Geometry: final body of the model. Coordinates: model frame, mm. Give positions to 0.01 mm unless a question says otherwise; leave off trailing zeros. Write each loop counter-clockwise with the first axis right and the second up, starting at its lowest first coordinate (ties: lowest second). Pieces come first, ordered by that corner, then holes. Notation, with made-up numbers: M 9.5,-10 L 23.5,-10 A13 cw 23.5,2 Z; hole C 22,-29 d9. An arc over 180 degrees is marked long. Answer as a JSON object with one key per item and string values.
from build123d import *

# Parameters (mm, degrees)
SKETCH_1_W          = 18
SKETCH_1_H          = 130
SKETCH_1_W_2        = 5
SKETCH_1_H_2        = 2
SKETCH_1_H_3        = 3
EXTRUDE_1_DEPTH     = 1.05
SKETCH_5_R          = 0.5
CUT_EXTRUDE_3_DEPTH = 69.625141166
SKETCH_2_W          = 1.05
SKETCH_2_H          = 25.1
CUT_EXTRUDE_1_DEPTH = 10
SKETCH_6_R          = 0.5
CUT_EXTRUDE_4_DEPTH = 69.625141166
CUT_EXTRUDE_5_DEPTH = 69.625141166
CUT_EXTRUDE_6_DEPTH = 69.625141166


with BuildPart() as part:
    # 草图1 → 凸台-拉伸1 (new, symmetric)
    with BuildSketch(Plane.XY):
        Rectangle(SKETCH_1_W, SKETCH_1_H)
        with Locations((-2.5, 66)):
            Rectangle(SKETCH_1_W_2, SKETCH_1_H_2)
        with Locations((2.5, 66)):
            Rectangle(SKETCH_1_W_2, SKETCH_1_H_2)
        with Locations((2.5, -66.5)):
            Rectangle(SKETCH_1_W_2, SKETCH_1_H_3)
        with Locations((-2.5, -66.5)):
            Rectangle(SKETCH_1_W_2, SKETCH_1_H_3)
    extrude(amount=EXTRUDE_1_DEPTH, both=True)

    # 草图5 → 切除-拉伸3 (cut, through all)
    with BuildSketch(Plane.XY.offset(1.05)):
        with Locations((5.353553391, 65.353553391)):
            Circle(SKETCH_5_R)
        with Locations((-5.353553391, 65.353553391)):
            Circle(SKETCH_5_R)
        with Locations((5.353553391, -65.353553391)):
            Circle(SKETCH_5_R)
        with Locations((-5.353553391, -65.353553391)):
            Circle(SKETCH_5_R)
    extrude(amount=-CUT_EXTRUDE_3_DEPTH, mode=Mode.SUBTRACT)

    # 草图2 → 切除-拉伸1 (cut)
    with BuildSketch(Plane.XY.offset(1.05)):
        with Locations((0.525, 37.5)):
            Rectangle(SKETCH_2_W, SKETCH_2_H)
        with Locations((-0.525, 37.5)):
            Rectangle(SKETCH_2_W, SKETCH_2_H)
        with Locations((0.525, -37.5)):
            Rectangle(SKETCH_2_W, SKETCH_2_H)
        with Locations((-0.525, -37.5)):
            Rectangle(SKETCH_2_W, SKETCH_2_H)
    extrude(amount=-CUT_EXTRUDE_1_DEPTH, mode=Mode.SUBTRACT)

    # 草图6 → 切除-拉伸4 (cut, through all)
    with BuildSketch(Plane.XY.offset(1.05)):
        with Locations((0.696446609, 49.696446609)):
            Circle(SKETCH_6_R)
        with Locations((-0.696446609, 49.696446609)):
            Circle(SKETCH_6_R)
        with Locations((0.696446609, 25.303553391)):
            Circle(SKETCH_6_R)
        with Locations((-0.696446609, 25.303553391)):
            Circle(SKETCH_6_R)
    cut_extrude_4 = extrude(amount=-CUT_EXTRUDE_4_DEPTH, mode=Mode.SUBTRACT)

    # 镜向1: 切除-拉伸4 across plane
    add(cut_extrude_4.mirror(Plane.ZX), mode=Mode.SUBTRACT)

    # 草图4 → 切除-拉伸5 (cut, through all)
    with BuildSketch(Plane.XY.offset(1.05)):
        with BuildLine():
            Line((6.2, 55), (6.2, 35))
            ThreePointArc((6.2, 35), (5, 33.8), (3.8, 35))
            Line((3.8, 35), (3.8, 55))
            ThreePointArc((3.8, 55), (5, 56.2), (6.2, 55))
        make_face()
        with BuildLine():
            Line((6.2, 25), (6.2, 5))
            ThreePointArc((6.2, 5), (5, 3.8), (3.8, 5))
            Line((3.8, 5), (3.8, 25))
            ThreePointArc((3.8, 25), (5, 26.2), (6.2, 25))
        make_face()
        with BuildLine():
            Line((6.2, -5), (6.2, -25))
            ThreePointArc((6.2, -25), (5, -26.2), (3.8, -25))
            Line((3.8, -25), (3.8, -5))
            ThreePointArc((3.8, -5), (5, -3.8), (6.2, -5))
        make_face()
        with BuildLine():
            Line((3.8, -55), (3.8, -35))
            ThreePointArc((3.8, -35), (5, -33.8), (6.2, -35))
            Line((6.2, -35), (6.2, -55))
            ThreePointArc((6.2, -55), (5, -56.2), (3.8, -55))
        make_face()
    cut_extrude_5 = extrude(amount=-CUT_EXTRUDE_5_DEPTH, mode=Mode.SUBTRACT)

    # 镜向2: 切除-拉伸5 across plane
    add(cut_extrude_5.mirror(Plane(origin=(0, 0, 0), x_dir=(0, 0, 1), z_dir=(1, 0, 0))), mode=Mode.SUBTRACT)

    # 草图7 → 切除-拉伸6 (cut, through all)
    with BuildSketch(Plane.XY.offset(1.05)):
        with BuildLine():
            Line((1.2, 62.05), (1.2, 55.05))
            ThreePointArc((1.2, 55.05), (0, 53.85), (-1.2, 55.05))
            Line((-1.2, 55.05), (-1.2, 62.05))
            ThreePointArc((-1.2, 62.05), (0, 63.25), (1.2, 62.05))
        make_face()
        with BuildLine():
            Line((1.2, 15), (1.2, -15))
            ThreePointArc((1.2, -15), (0, -16.2), (-1.2, -15))
            Line((-1.2, -15), (-1.2, 15))
            ThreePointArc((-1.2, 15), (0, 16.2), (1.2, 15))
        make_face()
        with BuildLine():
            Line((1.2, -55.05), (1.2, -62.05))
            ThreePointArc((1.2, -62.05), (0, -63.25), (-1.2, -62.05))
            Line((-1.2, -62.05), (-1.2, -55.05))
            ThreePointArc((-1.2, -55.05), (0, -53.85), (1.2, -55.05))
        make_face()
    extrude(amount=-CUT_EXTRUDE_6_DEPTH, mode=Mode.SUBTRACT)


solid = part.part
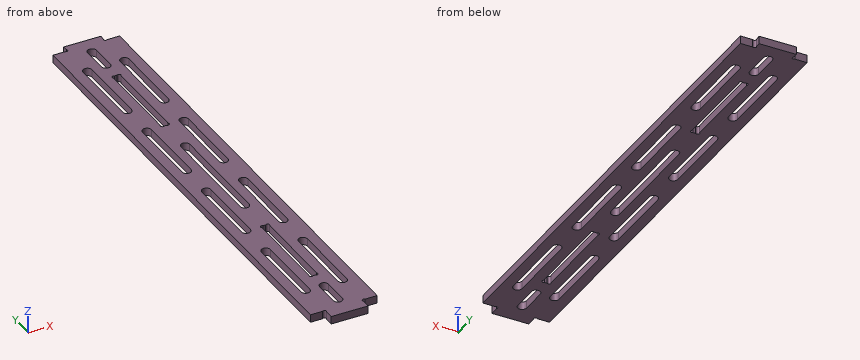
1) Cut plane D-D on z = -0.5. Give the number of separate pieces and of enclosed holes in the cut face, and give its area (3 significant figures).
Geometry check:
{"separate pieces": "1", "enclosed holes": "13", "area": "1,740 mm2"}
2) Line query: line 1 (X direction, y = -5.5, z = 0.35); line 2 (X direction, y = 50.5, z = 0.25); line 3 (X direction, y = 43, z = 0.25). Output: solid intervals per line, ascending. Write a range as from..to.
Geometry check:
{"line 1": "x = -9..-6.2, -3.8..-1.2, 1.2..3.8, 6.2..9", "line 2": "x = -9..-6.2, -3.8..3.8, 6.2..9", "line 3": "x = -9..-6.2, -3.8..-1.05, 1.05..3.8, 6.2..9"}
3) Contact query for flat-ended pins moving along their axis: P1, Ø0.6, axis at x = 7, z = -0.5, coming from the -Y side; P2, Ø1, axis at y = 66, z = 0.5, coming from the -X side; P3, Ø0.6, axis at y = -67, z = 0.5, coming from the +X side. Output: stop coordinate, or through.
Geometry check:
{"P1": "stops at y = -65", "P2": "stops at x = -5", "P3": "stops at x = 5"}
4) Cut plane B-B on y = -28. Return loops of the section in (x, z), and give its area (3 significant figures).
Geometry check:
{"outline": "M -9,-1.05 L -1.05,-1.05 L -1.05,1.05 L -9,1.05 Z; M 1.05,-1.05 L 9,-1.05 L 9,1.05 L 1.05,1.05 Z", "area": "33.4 mm2"}
5) Cut plane C-C on y = 8.5. Return loops of the section in (x, z), and give its area (3 significant figures).
Geometry check:
{"outline": "M -9,-1.05 L -6.2,-1.05 L -6.2,1.05 L -9,1.05 Z; M -3.8,-1.05 L -1.2,-1.05 L -1.2,1.05 L -3.8,1.05 Z; M 1.2,-1.05 L 3.8,-1.05 L 3.8,1.05 L 1.2,1.05 Z; M 6.2,-1.05 L 9,-1.05 L 9,1.05 L 6.2,1.05 Z", "area": "22.7 mm2"}
6) Cut plane A-A on y = -42. Return loops of the section in (x, z).
Geometry check:
{"outline": "M -9,-1.05 L -6.2,-1.05 L -6.2,1.05 L -9,1.05 Z; M -3.8,-1.05 L -1.05,-1.05 L -1.05,1.05 L -3.8,1.05 Z; M 1.05,-1.05 L 3.8,-1.05 L 3.8,1.05 L 1.05,1.05 Z; M 6.2,-1.05 L 9,-1.05 L 9,1.05 L 6.2,1.05 Z"}
